Geometry check sheet. Reference: the model listing, model coordinates, mm. Face numbers are marked on the shaded views. A direction names the side the tool comes from. Round coordinates to 2 decimals unless told otherwise and drop trailing zeros. Write each loop counter-clockwise with the first axis right and the second up, starting at its lowest first coordinate (ties: lowest second). Pieces come first, ordered by that corner, then holes.
Item 1: Draft check along X on the marked faces 4, 5, 6 and 7. Enter one of: pulls with the +X half, pulls with the -X half, needs draft (parallel to the pull), parting line crosses it, or undercut.
Item 2: Cross-section at C-C (y = 0). Enter the section's corners in (x, z), then the cut area to 3 significant figures.
Item 3: Cross-section at D-D (x = -7). Enter the section's corners in (y, z).
Item 4: Depth check by flat-ended pin: P1, Ø5, axis at x = 4, z = 2, coming from the +Y side; P2, Ø8, axis at x = 24, z = 6.5, coming from the +Y side; P3, Ø1.5, axis at x = -22, y = -2, coming from the +Z side. Enter the tip coordinate at first touch or a pass-through.
Item 5: Scan lines: probe 1 along Z at (x, y) = (2.5, -2); probe 2 along Y at (x, z) = (-0.5, 41.5); probe 3 along Z at (x, y) = (14, -4). Record each from-to range of solid material in increasing order.
Item 6: Access from +Z, -Z, +X, -X, +Y, -Y to the whole of each face (thin tool, end or side, straight path). Record for the marked faces 1, 2 and 3.
from build123d import *

# Parameters (mm, degrees)
BOSS_EXTRUDE1_DEPTH = 6.35
FILLET1_R           = 25.4
SKETCH3_R           = 3.175
BOSS_EXTRUDE2_DEPTH = 9.525
FILLET2_R           = 3.175
SKETCH4_R           = 7.9375
BOSS_EXTRUDE3_DEPTH = 38.1


with BuildPart() as part:
    # Sketch2 → Boss-Extrude1 (new body)
    with BuildSketch(Plane.XY):
        with BuildLine():
            Line((-15.859729928, -20.155141971), (0, -10.998522628))
            Line((0, -10.998522628), (15.859729928, -20.155141971))
            ThreePointArc((15.859729928, -20.155141971), (28.871121899, -16.66875), (25.384729928, -3.657358029))
            Line((25.384729928, -3.657358029), (9.525, 5.499261314))
            Line((9.525, 5.499261314), (9.525, 23.8125))
            ThreePointArc((9.525, 23.8125), (0, 33.3375), (-9.525, 23.8125))
            Line((-9.525, 23.8125), (-9.525, 5.499261314))
            Line((-9.525, 5.499261314), (-25.384729928, -3.657358029))
            ThreePointArc((-25.384729928, -3.657358029), (-28.871121899, -16.66875), (-15.859729928, -20.155141971))
        make_face()
    extrude(amount=BOSS_EXTRUDE1_DEPTH)

    # Fillet1
    fillet1_edges = [part.edges().sort_by_distance(p)[0] for p in [
        (-9.525, 5.499261314, 3.175),
        (9.525, 5.499261314, 3.175),
        (0, -10.998522628, 3.175),
    ]]
    fillet(fillet1_edges, radius=FILLET1_R)

    # Sketch3 → Boss-Extrude2 (add)
    with BuildSketch(Plane(origin=(0, 0, 0), x_dir=(-1, 0, 0), z_dir=(0, 0, -1))):
        with Locations(Location((0, 23.8125, 0), (0, 0, 180))):
            Circle(SKETCH3_R)
        with Locations(Location((20.622229928, -11.90625, 0), (0, 0, 180))):
            Circle(SKETCH3_R)
        with Locations(Location((-20.622229928, -11.90625, 0), (0, 0, 180))):
            Circle(SKETCH3_R)
    extrude(amount=BOSS_EXTRUDE2_DEPTH)

    # Fillet2
    fillet2_edges = [part.edges().sort_by_distance(p)[0] for p in [
        (-3.175, 23.8125, -9.525),
        (-23.797229928, -11.90625, -9.525),
        (17.447229928, -11.90625, -9.525),
    ]]
    fillet(fillet2_edges, radius=FILLET2_R)

    # Sketch4 → Boss-Extrude3 (add)
    with BuildSketch(Plane.XY.offset(6.35)):
        with Locations(Location((0, 0, 0), (0, 0, 180))):
            Circle(SKETCH4_R)
    extrude(amount=BOSS_EXTRUDE3_DEPTH)


solid = part.part
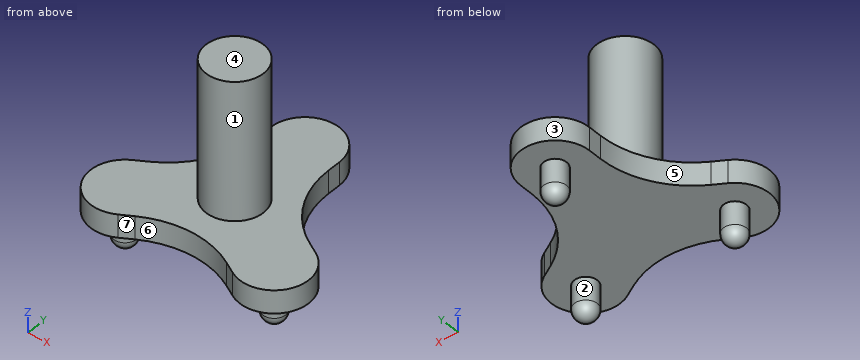
Resolved:
1. face 4: needs draft
1. face 5: pulls with the -X half
1. face 6: undercut
1. face 7: undercut
2. outline: (-19.48, 0) - (19.48, 0) - (19.48, 6.35) - (7.94, 6.35) - (7.94, 44.45) - (-7.94, 44.45) - (-7.94, 6.35) - (-19.48, 6.35) - close
2. area: 852 mm2
3. outline: (-15.91, 0) - (30.27, 0) - (30.27, 6.35) - (3.74, 6.35) - (3.74, 44.45) - (-3.74, 44.45) - (-3.74, 6.35) - (-15.91, 6.35) - close
4. P1: stops at y = 33.22
4. P2: stops at y = -0.39
4. P3: stops at z = 6.35
5. probe 1: z = 0 to 44.45
5. probe 2: y = -7.92 to 7.92
5. probe 3: z = 0 to 6.35
6. face 1: +Z
6. face 2: -Z
6. face 3: +Z, -Z, +Y
